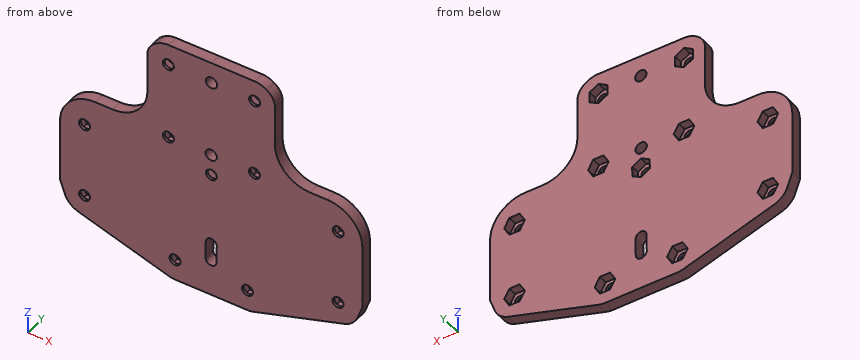
```python
from build123d import *

# Parameters (mm, degrees)
SKETCH2_R          = 3.15
SKETCH2_R_2        = 3.25
SKETCH2_R_3        = 3.1
MAINPLATE_DEPTH    = 6.5
PRESSFITNUTS_DEPTH = 5
CUT_EXTRUDE2_DEPTH = 6.5
FILLET2_R          = 10


with BuildPart() as part:
    # Sketch2 → MainPlate (new body)
    with BuildSketch(Plane(origin=(0, 0, 0), x_dir=(1, 0, 0), z_dir=(0, 1, 0))):
        with BuildLine():
            Line((24.899900609, -92.429929219), (0.2, -92.5))
            Line((0.2, -92.5), (-24.5, -92.5))
            ThreePointArc((-24.5, -92.5), (-27.871368271, -92.016678166), (-30.971160559, -90.605645997))
            Line((-30.971160559, -90.605645997), (-99.683475736, -46.605645997))
            ThreePointArc((-99.683475736, -46.605645997), (-104.578950448, -40.347025165), (-104.490786491, -32.401697323))
            Line((-104.490786491, -32.401697323), (-83.778471314, 24.598302677))
            ThreePointArc((-83.778471314, 24.598302677), (-80.773721892, 29.191692934), (-76.037940173, 31.966602781))
            Line((-76.037940173, 31.966602781), (-24.911380811, 47.741345462))
            ThreePointArc((-24.911380811, 47.741345462), (-22.845839779, 48.308813352), (-20.712315177, 48.5))
            Line((-20.712315177, 48.5), (0, 48.5))
            Line((0, 48.5), (20.712231832, 48.558758223))
            ThreePointArc((20.712231832, 48.558758223), (22.846290221, 48.373624884), (24.913432777, 47.812018957))
            Line((24.913432777, 47.812018957), (76.084537362, 32.182379345))
            ThreePointArc((76.084537362, 32.182379345), (80.828172093, 29.420915478), (83.845940292, 24.836067799))
            Line((83.845940292, 24.836067799), (104.719873926, -32.104944614))
            ThreePointArc((104.719873926, -32.104944614), (104.830577421, -40.049990373), (99.952877324, -46.322473865))
            Line((99.952877324, -46.322473865), (31.365661085, -90.517224974))
            ThreePointArc((31.365661085, -90.517224974), (28.26988419, -91.937045184), (24.899900609, -92.429929219))
        make_face()
        with Locations(Location((-72.5, 20.5, 0), (0, 0, 90))):
            Circle(SKETCH2_R, mode=Mode.SUBTRACT)
        with Locations(Location((-20.712315177, 36.5, 0), (0, 0, 90))):
            Circle(SKETCH2_R, mode=Mode.SUBTRACT)
        with Locations(Location((-93.212315177, -36.5, 0), (0, 0, 90))):
            Circle(SKETCH2_R, mode=Mode.SUBTRACT)
        with Locations(Location((-58.856157589, -58.5, 0), (0, 0, 90))):
            Circle(SKETCH2_R, mode=Mode.SUBTRACT)
        with Locations(Location((-24.5, -80.5, 0), (0, 0, 90))):
            Circle(SKETCH2_R, mode=Mode.SUBTRACT)
        with Locations(Location((-24.5, -36.5, 0), (0, 0, 90))):
            Circle(SKETCH2_R, mode=Mode.SUBTRACT)
        with Locations(Location((-72.5, -22.5, 0), (0, 0, 90))):
            Circle(SKETCH2_R, mode=Mode.SUBTRACT)
        with Locations(Location((24.74103568, -36.430154559, 0), (0, 0, 90))):
            Circle(SKETCH2_R, mode=Mode.SUBTRACT)
        with Locations(Location((24.865858124, -80.429977506, 0), (0, 0, 90))):
            Circle(SKETCH2_R, mode=Mode.SUBTRACT)
        with Locations(Location((59.159466244, -58.332601952, 0), (0, 0, 90))):
            Circle(SKETCH2_R, mode=Mode.SUBTRACT)
        with Locations(Location((93.453074364, -36.235226398, 0), (0, 0, 90))):
            Circle(SKETCH2_R, mode=Mode.SUBTRACT)
        with Locations(Location((72.701126299, -22.294040956, 0), (0, 0, 90))):
            Circle(SKETCH2_R, mode=Mode.SUBTRACT)
        with Locations(Location((72.579140729, 20.705786015, 0), (0, 0, 90))):
            Circle(SKETCH2_R, mode=Mode.SUBTRACT)
        with Locations(Location((20.746274317, 36.55880651, 0), (0, 0, 90))):
            Circle(SKETCH2_R, mode=Mode.SUBTRACT)
        with Locations(Location((0, -36.5, 0), (0, 0, 90))):
            Circle(SKETCH2_R_2, mode=Mode.SUBTRACT)
        with Locations(Location((0.182929062, -80.464988753, 0), (0, 0, 90))):
            Circle(SKETCH2_R_2, mode=Mode.SUBTRACT)
        with Locations(Location((0.103546099, -24.5, 0), (0, 0, 90))):
            Circle(SKETCH2_R_3, mode=Mode.SUBTRACT)
        with BuildLine():
            Line((3.105906565, 27.527701056), (3.193849827, 17.527701056))
            ThreePointArc((3.193849827, 17.527701056), (0.071672688, 14.350121804), (-3.105906565, 17.472298944))
            Line((-3.105906565, 17.472298944), (-3.193849827, 27.472298944))
            ThreePointArc((-3.193849827, 27.472298944), (-0.071672688, 30.649878196), (3.105906565, 27.527701056))
        make_face(mode=Mode.SUBTRACT)
    extrude(amount=MAINPLATE_DEPTH)

    # Sketch8 → PressFitNuts (cut)
    with BuildSketch(Plane(origin=(0, 6.5, 0), x_dir=(1, 0, 0), z_dir=(0, 1, 0))):
        Polygon((-4.835460238, -27.48990798), (0.223379197, -30.272258948), (5.162385534, -27.282350968), (5.042552437, -21.51009202), (-0.016286998, -18.727741052), (-4.955293335, -21.717649032), align=None)
        Polygon((-18.582159741, -36.5), (-21.54107987, -31.375), (-27.45892013, -31.375), (-30.417840259, -36.5), (-27.45892013, -41.625), (-21.54107987, -41.625), align=None)
        Polygon((-66.582159741, -22.5), (-69.54107987, -17.375), (-75.45892013, -17.375), (-78.417840259, -22.5), (-75.45892013, -27.625), (-69.54107987, -27.625), align=None)
        Polygon((-66.582159741, 20.5), (-69.54107987, 25.625), (-75.45892013, 25.625), (-78.417840259, 20.5), (-75.45892013, 15.375), (-69.54107987, 15.375), align=None)
        Polygon((-87.294474918, -36.5), (-90.253395048, -31.375), (-96.171235307, -31.375), (-99.130155436, -36.5), (-96.171235307, -41.625), (-90.253395048, -41.625), align=None)
        Polygon((-52.938317329, -58.5), (-55.897237459, -53.375), (-61.815077718, -53.375), (-64.773997848, -58.5), (-61.815077718, -63.625), (-55.897237459, -63.625), align=None)
        Polygon((-24.5, -74.582159741), (-29.625, -77.54107987), (-29.625, -83.45892013), (-24.5, -86.417840259), (-19.375, -83.45892013), (-19.375, -77.54107987), align=None)
        Polygon((-14.794474918, 36.5), (-17.753395048, 41.625), (-23.671235307, 41.625), (-26.630155436, 36.5), (-23.671235307, 31.375), (-17.753395048, 31.375), align=None)
        Polygon((17.753395048, 31.375), (14.794474918, 36.5), (17.753395048, 41.625), (23.671235307, 41.625), (26.630155436, 36.5), (23.671235307, 31.375), align=None)
        Polygon((19.375, -77.54107987), (24.5, -74.582159741), (29.625, -77.54107987), (29.625, -83.45892013), (24.5, -86.417840259), (19.375, -83.45892013), align=None)
        Polygon((55.897237459, -63.625), (52.938317329, -58.5), (55.897237459, -53.375), (61.815077718, -53.375), (64.773997848, -58.5), (61.815077718, -63.625), align=None)
        Polygon((90.253395048, -41.625), (87.294474918, -36.5), (90.253395048, -31.375), (96.171235307, -31.375), (99.130155436, -36.5), (96.171235307, -41.625), align=None)
        Polygon((69.54107987, 15.375), (66.582159741, 20.5), (69.54107987, 25.625), (75.45892013, 25.625), (78.417840259, 20.5), (75.45892013, 15.375), align=None)
        Polygon((69.54107987, -27.625), (66.582159741, -22.5), (69.54107987, -17.375), (75.45892013, -17.375), (78.417840259, -22.5), (75.45892013, -27.625), align=None)
        Polygon((21.54107987, -41.625), (18.582159741, -36.5), (21.54107987, -31.375), (27.45892013, -31.375), (30.417840259, -36.5), (27.45892013, -41.625), align=None)
    extrude(amount=-PRESSFITNUTS_DEPTH, mode=Mode.SUBTRACT)

    # Sketch11 → Cut-Extrude2 (cut)
    with BuildSketch(Plane(origin=(0, 0, 0), x_dir=(1, 0, 0), z_dir=(0, 1, 0))):
        with BuildLine():
            Line((-111.9, 4.5), (-111.9, -116.15))
            Line((-111.9, -116.15), (-86.5, -116.15))
            Line((-86.5, -116.15), (-36.5, -116.15))
            Line((-36.5, -116.15), (-36.5, -59))
            ThreePointArc((-36.5, -59), (-42.357864376, -44.857864376), (-56.5, -39))
            Line((-56.5, -39), (-66.5, -39))
            ThreePointArc((-66.5, -39), (-80.642135624, -33.142135624), (-86.5, -19))
            Line((-86.5, -19), (-86.5, 4.5))
            Line((-86.5, 4.5), (-86.5, 44.576396133))
            Line((-86.5, 44.576396133), (-111.9, 44.576396133))
            Line((-111.9, 44.576396133), (-111.9, 4.5))
        make_face()
        with BuildLine():
            Line((86.5, 4.5), (86.5, 44.576396133))
            Line((86.5, 44.576396133), (111.9, 44.576396133))
            Line((111.9, 44.576396133), (111.9, 4.5))
            Line((111.9, 4.5), (111.9, -116.15))
            Line((111.9, -116.15), (86.5, -116.15))
            Line((86.5, -116.15), (36.5, -116.15))
            Line((36.5, -116.15), (36.5, -59))
            ThreePointArc((36.5, -59), (42.357864376, -44.857864376), (56.5, -39))
            Line((56.5, -39), (66.5, -39))
            ThreePointArc((66.5, -39), (80.642135624, -33.142135624), (86.5, -19))
            Line((86.5, -19), (86.5, 4.5))
        make_face()
    extrude(amount=CUT_EXTRUDE2_DEPTH, mode=Mode.SUBTRACT)

    # Fillet2
    fillet2_edges = [part.edges().sort_by_distance(p)[0] for p in [
        (36.5, 3.25, 87.208870401),
        (-36.5, 3.25, 87.065248111),
    ]]
    fillet(fillet2_edges, radius=FILLET2_R)


solid = part.part
```
For this review, take the finished solid that the model builds, in its own axes (mm). Round coordinates to 2 decimals unless told otherwise and drop trailing zeros. Write each loop counter-clockwise with the first axis right and the second up, starting at its lowest first coordinate (ties: lowest second). Pieces come first, ordered by that corner, then holes. Notation, with made-up numbers: (63.5, 74) - (84.5, 74) arc R3 cw to (84.5, 78) - close; hole circle Ø8 at (-27, -29.75). An arc over 180 degrees is marked (long way). Write each question's results on one line, items separated by ' | '.
Item 1: For pin 1 (2 mm diameter, centred on x = -6.5, y = 2.5, fed in from -Z); pin 2 (1 mm diameter, centred on y = 5, z = 47.5, fed in from +X); pin 3 (1 mm diameter, centred on x = 58, y = 5, fed in from +Z), all flat-tipped, find the tip position at first contact; note any pin that passes through.
Calculated:
pin 1: stops at z = -48.5 | pin 2: stops at x = 40.5 | pin 3: stops at z = 39
Item 2: Take a section at A-A on x = -72.5. State the section outline as (y, z) points (3 decimals).
Calculated:
outline: (0, -33.058) - (6.5, -33.058) - (6.5, -25.625) - (1.5, -25.625) - (1.5, -23.65) - (0, -23.65) - close; (0, -17.35) - (1.5, -17.35) - (1.5, -15.375) - (6.5, -15.375) - (6.5, 17.375) - (1.5, 17.375) - (1.5, 19.35) - (0, 19.35) - close; (0, 25.65) - (1.5, 25.65) - (1.5, 27.625) - (6.5, 27.625) - (6.5, 38.079) - (0, 38.079) - close
Item 3: Take a section at B-B on y = 3. Count the separate pieces of the cut face and the enclosed holes in it, then the cut area to 3 significant figures.
Calculated:
separate pieces: 1 | enclosed holes: 14 | area: 16,500 mm^2
Item 4: To check wall thickness, follow line 1 along X through (y, z) = (1.15, 36.5); line 2 along Z through (x, y) = (-2, 0.5); line 3 along X through (y, z) = (4.5, 36.5). State the ranges of each line that lie inside material, in increasing order. Write a range as from..to.
Calculated:
line 1: x = -76.18..-27.65, -21.35..-3.25, 3.25..21.59, 27.89..76.18 | line 2: z = -48.5..-29.97, -15.1..22.22, 26.78..33.94, 39.06..78.06, 82.87..92.5 | line 3: x = -76.18..-30.42, -18.58..-3.25, 3.25..18.58, 30.42..76.18
Item 5: Take a section at C-C on x = -54.5. State the section outline as (y, z) points, then the cut area to 3 significant figures.
Calculated:
outline: (0, -38.61) - (6.5, -38.61) - (6.5, 39.1) - (0, 39.1) - close | area: 505 mm^2
